Geometry: final body of the model. Coordinates: model frame, mm. Round coordinates to 2 decimals unless told otherwise and drop trailing zeros. Loops run counter-clockwise (first coordinate to the right, second up) from the corner with the lowest first, then second, coordinate; pieces in that order, holes last. Notation, with made-up numbers: (56.25, 2.5) - (62.25, 2.5) arc R33 cw to (62.25, 36.5) - close; hole circle Ø11 at (-39.5, 0.5). An arc over 180 degrees is marked (long way). Answer as a JSON object with one key per item and string values. Group by question number.
Item 1: Line query: line 1 (Z direction, x = 0, y = 0.1); line 2 (X direction, y = -0.1, z = -3); line 3 (Z direction, x = -0.45, y = -0.05). Output: solid intervals per line, ascending.
Item 2: Section C-C (z = -4.25). Return the cut outline in (x, y).
Item 3: Draft query along Z for faces 1 (the face through (0, -0.25, -1)), 2 (the face through (-0.323, -0.004, 3.606)), 3 (the face through (0, 0, 4.5)). Return one class per face: released by +Z, released by -Z, zero draft, split by the parting line, or undercut.
Item 4: Section B-B (y = -0.05). Return the cut outline in (x, z).
Item 5: Section A-A (x = 0). Return the cut outline in (y, z).
```python
from build123d import *

# Parameters (mm, degrees)
SKETCH_R  = 0.6
PAD_DEPTH = 0.25


with BuildPart() as part:
    # Sketch → Pad (new body, symmetric)
    with BuildSketch(Plane(origin=(0, 0, 0), x_dir=(-1, 0, 0), z_dir=(0, 1, 0))):
        with BuildLine():
            Line((-1.4, 3.1), (-1.4, 0))
            Line((-1.4, 0), (-0.7, 0))
            Line((-0.7, 0), (-0.7, -6.1))
            ThreePointArc((-0.7, -6.1), (0, -6.8), (0.7, -6.1))
            Line((0.7, 0), (0.7, -6.1))
            Line((0.7, 0), (1.4, 0))
            Line((1.4, 0), (1.4, 3.1))
            ThreePointArc((1.4, 3.1), (0, 4.5), (-1.4, 3.1))
        make_face()
        with Locations((0, 3.1)):
            Circle(SKETCH_R, mode=Mode.SUBTRACT)
    extrude(amount=PAD_DEPTH, both=True)


solid = part.part
```
Values:
{
 "1": {"line 1": "z = -6.8 to 2.5, 3.7 to 4.5", "line 2": "x = -0.7 to 0.7", "line 3": "z = -6.64 to 2.7, 3.5 to 4.43"},
 "2": {"outline": "(-0.7, -0.25) - (0.7, -0.25) - (0.7, 0.25) - (-0.7, 0.25) - close"},
 "3": {"face 1": "zero draft", "face 2": "undercut", "face 3": "released by +Z"},
 "4": {"outline": "(-1.4, 0) - (-0.7, 0) - (-0.7, -6.1) arc R0.7 ccw to (0.7, -6.1) - (0.7, 0) - (1.4, 0) - (1.4, 3.1) arc R1.4 ccw to (-1.4, 3.1) - close; hole circle Ø1.2 at (0, 3.1)"},
 "5": {"outline": "(-0.25, -6.8) - (0.25, -6.8) - (0.25, 2.5) - (-0.25, 2.5) - close; (-0.25, 3.7) - (0.25, 3.7) - (0.25, 4.5) - (-0.25, 4.5) - close"}
}
